from build123d import *

# Parameters (mm, degrees)
F0_R     = 9.5
F1_DEPTH = 160
F2_W     = 37.5
F2_H     = 20
F3_DEPTH = 30
F4_R     = 7.5
F5_DEPTH = 1000
F7_R     = 25.75
F7_R_2   = 25
F8_DEPTH = 12.5
F9_DEPTH = 500


with BuildPart() as f1:
    # F0 (on Front) → F1 (new body)
    with BuildSketch(Plane.XZ):
        Circle(F0_R)
    extrude(amount=-F1_DEPTH)

    # F2 (on Front) → F3 (cut)
    with BuildSketch(Plane.XZ):
        Rectangle(F2_W, F2_H)
    extrude(amount=F3_DEPTH, mode=Mode.SUBTRACT)

    # F4 (on Top) → F5 (cut, symmetric)
    with BuildSketch(Plane.XY):
        with Locations((0, 8.5)):
            Circle(F4_R)
    extrude(amount=F5_DEPTH, both=True, mode=Mode.SUBTRACT)

    # F6: F1 across face


with BuildPart() as f1_1:
    add(f1.part)
    add(f1.part.mirror(Plane(origin=(0, 160, 0), x_dir=(1, 0, 0), z_dir=(0, 1, 0))))

    # F7 (on Top) → F8 (join, symmetric)
    with BuildSketch(Plane.XY):
        with Locations((0, 320)):
            Circle(F7_R)
        with Locations((0, 320)):
            Circle(F7_R_2, mode=Mode.SUBTRACT)
    extrude(amount=F8_DEPTH, both=True)

    # F7 (on Top) → F9 (cut, symmetric)
    with BuildSketch(Plane.XY):
        with Locations((0, 320)):
            Circle(F7_R_2)
    extrude(amount=F9_DEPTH, both=True, mode=Mode.SUBTRACT)


solid = f1_1.part
Geometry: final body of the model. Coordinates: model frame, mm. Give positions to 0.01 mm unless a question says otherwise; leave off trailing zeros. Loops run counter-clockwise (first coordinate to the right, second up) from the corner with the lowest first, then second, coordinate; pieces in that order, holes last. Notation, with made-up numbers: M 80,39.25 L 104,39.25 A13 cw 104,59.25 Z; hole C 87.5,83.25 d2. An arc over 180 degrees is marked long. Put each result on its own line as item: value. Start each with the question number.
1) Ray query, line 1 along Y through (x, z) = (0, 2.25); line 2 along X through (y, z) = (8.5, -0.25); line 3 along Y through (x, z) = (-2, 4.75). Return the intervals inside material, ascending.
2) Cut plane B-B (y = 320). Output: boundary loops of the cut face in (x, z), then the cut area to 3 significant figures.
3) Cut plane A-A (x = 0). Output: boundary loops of the cut face in (y, z).
4) Cut plane D-D (x = -17). Output: boundary loops of the cut face in (y, z), then the cut area to 3 significant figures.
5) Pull-direction query (X, two-part tool) for faces 1 (the cylindrical face through (13.843, 341.712, 0.175)), 2 (the flat face through (0, 0, 0)), 3 (the cylindrical face through (6.93, 5.63, 0.13)); classes: pulls with the +X half, pulls with the -X half, needs draft (parallel to the pull), parting line crosses it, or undercut.
6) Contact query for flat-ended pins moving along their axis: pin 1 (6 mm diameter, centred on y = 225.5, z = -9.5, fed in from -X); pin 2 (2 mm diameter, centred on x = 19, z = 6, fed in from -Y); pin 3 (19.5 mm diameter, centred on x = 0, y = 8.5, fed in from +Z). Output: stop coordinate, or through.
7) Cut plane C-C (z = 0). Output: boundary loops of the cut face in (x, y), then the cut area to 3 significant figures.
Verdict:
1. line 1: 0 to 1, 16 to 295, 345 to 345.75
1. line 2: -9.5 to -7.5, 7.5 to 9.5
1. line 3: 0 to 1.27, 15.73 to 295.08, 344.92 to 345.67
2. outline: M -25.75,-12.5 L -25,-12.5 L -25,12.5 L -25.75,12.5 Z; M 25,-12.5 L 25.75,-12.5 L 25.75,12.5 L 25,12.5 Z
2. area: 37.5 mm2
3. outline: M 0,-9.5 L 1,-9.5 L 1,9.5 L 0,9.5 Z; M 16,-9.5 L 294.25,-9.5 L 294.25,-12.5 L 295,-12.5 L 295,12.5 L 294.25,12.5 L 294.25,9.5 L 16,9.5 Z; M 345,-12.5 L 345.75,-12.5 L 345.75,12.5 L 345,12.5 Z
4. outline: M 300.66,-12.5 L 301.67,-12.5 L 301.67,12.5 L 300.66,12.5 Z; M 338.33,-12.5 L 339.34,-12.5 L 339.34,12.5 L 338.33,12.5 Z
4. area: 50.5 mm2
5. face 1: parting line crosses it
5. face 2: needs draft
5. face 3: undercut
6. pin 1: x = -6.93
6. pin 2: y = 301.59
6. pin 3: z = 9.5
7. outline: M -9.5,0 L 9.5,0 L 9.5,296.07 A25.75 ccw long -9.5,296.07 Z; hole C 0,320 d50; hole C 0,8.5 d15
7. area: 5,540 mm2
